Autodesk Inventor part; units mm, degrees
ref_plane "YZ Plane" through (0, 0, 0) normal (1, 0, 0) x (0, 1, 0)
ref_plane "XZ Plane" through (0, 0, 0) normal (0, 1, 0) x (-1, 0, 0)
ref_plane "XY Plane" through (0, 0, 0) normal (0, 0, 1) x (1, 0, 0)
sketch "Szkic1" plane through (0, 0, 0) normal (0, 0, 1) x (1, 0, 0)
  line L0 (-25.2071, 0) -> (82.5929, 0)
  line L1 (0, -16) -> (0, 96)
  line L2 (0, 0) -> (0, 6) construction
  line L3 (0, 6) -> (-4.1, 6)
  line L4 (-4.1, 6) -> (-4.8071, 5.2929)
  line L5 (-4.1, 6) -> (-3.1, 6) construction
  line L6 (0, 0) -> (-4.8071, 0) construction
  line L7 (-4.8071, 0) -> (-4.8071, 3) construction
  line L8 (-4.8071, 3) -> (-4.8071, 5.2929)
  line L9 (-4.8071, 3) -> (-9.8071, 3)
  line L10 (-9.8071, 3) -> (-9.8071, 80)
  line L11 (-9.8071, 3) -> (67.1929, 3) construction
  line L12 (-9.8071, 80) -> (0, 80)
  line L13 (0, 80) -> (0, 6)
  dimension "d0" = 6
  dimension "d1" = 4.1
  dimension "d5" = 1
  dimension "d6" = 135
  dimension "d7" = 3
  dimension "d8" = 5
  dimension "d9" = 77
  dimension "d10" = 90
revolve "Obrót1" add sketch "Szkic1" angle 360 about axis through (-10, 0, 0) along (1, 0, 0)
sketch "Szkic2" plane through (-9.8071, 0, 0) normal (-1, 0, 0) x (0, 0, 1)
  line L0 (0, 0) -> (11, 0) construction
  circle A0 centre (11, 0) radius 1.55
  circle A1 centre (7.7782, 7.7782) radius 1.55
  circle A2 centre (0, 11) radius 1.55
  circle A3 centre (-7.7782, 7.7782) radius 1.55
  circle A4 centre (-11, 0) radius 1.55
  circle A5 centre (-7.7782, -7.7782) radius 1.55
  circle A6 centre (0, -11) radius 1.55
  circle A7 centre (7.7782, -7.7782) radius 1.55
  circle A8 centre (0, 0) radius 14
  circle A9 centre (0, 0) radius 5.05
  line L1 (5.8312, 0) -> (2.9156, -5.05)
  line L2 (2.9156, 5.05) -> (5.8312, 0)
  line L3 (-2.9156, 5.05) -> (2.9156, 5.05)
  line L4 (-5.8312, 0) -> (-2.9156, 5.05)
  line L5 (-2.9156, -5.05) -> (-5.8312, 0)
  line L6 (2.9156, -5.05) -> (-2.9156, -5.05)
  point P0 (0, -5.05)
  dimension "d21" = 10.1
  dimension "d12" = 11
  dimension "d13" = 3.1
  dimension "d16" = 360
  dimension "d20" = 28
  dimension "d26" = 360
extrude "Wyciągnięcie proste1" cut sketch "Szkic2" against normal through all contours A0 | A1 | A2 | A3 | A4 | A5 | A6 | A7
extrude "Wyciągnięcie proste2" add sketch "Szkic2" along normal blind 10
fillet "Zaokrąglenie1" radius 10 1 edges at (-9.8071, 0, -14)
properties part number "uMule-kolo_napędowe"
Verification items for the finished model (mm, model axes). A direction names the side the tool comes from. Coordinates: 2 decimals unless noted, no trailing zeros. Write each loop counter-clockwise with the first axis right and the second up, starting at its lowest first coordinate (ties: lowest second). Pieces come first, ordered by that corner, then holes. Notation, with made-up numbers: M 34,46 L 89,46 A28 cw 89,77 Z; hole C 23.25,80 d2. An arc over 180 degrees is marked long. One line per item, written item: value.
Item 1: Gauge pin test, flat ends, axial feed: pin 1 Ø2.5 at (y, z) = (-7.78, 7.78) entering from +X; pin 2 Ø1.7 at (x, z) = (-17, -1) entering from +Y; pin 3 Ø8 at (y, z) = (0, 0) entering from -X; pin 4 Ø1.5 at (x, z) = (-8.5, -45.5) entering from -Y. Record the tip position at first contact, or that the pin passes through.
Check sheet entries:
pin 1: passes through
pin 2: stops at y = 14.66
pin 3: stops at x = -9.81
pin 4: stops at y = -66.31
Item 2: Access from +Z, -Z, +X, -X, +Y, -Y to the whole of each face (thin tool, end or side, straight path). Record for faces 4 (the flat face through (0, 17, 1)), 5 (the cylindrical face through (-2, -6, 0)), 6 (the flat face through (-9.807, 17, 19)).
Check sheet entries:
face 4: +Z, -Z, +X, +Y, -Y
face 5: +X
face 6: -X
Item 3: Mould release check, pull along Z, two halves, no side actions. Record for faces 1 (the flat face through (-19.807, -6, 0)), 2 (the flat face through (-15, 5.05, 0)), 3 (the cylindrical face through (-4.83, -17.34, -78.1)): pulls with the +Z half, pulls with the -Z half, needs draft (parallel to the pull), parting line crosses it, or undercut.
Check sheet entries:
face 1: needs draft
face 2: undercut
face 3: parting line crosses it
Item 4: Section check B-B, the plane y = 64. Record the boundary of the cut face in (x, z).
Check sheet entries:
outline: M -9.81,-48 L 0,-48 L 0,48 L -9.81,48 Z
Item 5: Scan lines: line 1 along Z through (x, y) = (-13.25, -6.5); line 2 along X through (y, z) = (17.5, -33.5); line 3 along Y through (x, z) = (-12, 0). Record each from-to range of solid material in increasing order.
Check sheet entries:
line 1: z = -15.11 to -8.65, -6.9 to 6.9, 8.65 to 15.11
line 2: x = -9.81 to 0
line 3: y = -17.75 to -12.55, -9.45 to -5.05, 5.05 to 9.45, 12.55 to 17.75
Item 6: Section check A-A, the plane x = -14.5. State how many separate pieces and enclosed holes the cut face has, plus the area to 3 significant figures.
Check sheet entries:
separate pieces: 1
enclosed holes: 9
area: 608 mm^2
Item 7: Section check C-C, the plane z = 28. Record the boundary of the cut face in (x, y), plus the area to 3 significant figures.
Check sheet entries:
outline: M -9.81,-74.94 L 0,-74.94 L 0,74.94 L -9.81,74.94 Z
area: 1,470 mm^2
